Source: three-view drawing plus pictorial views. Frame: mm from the lowest corner of the part. A direction names the side the tool comes from. Coordinates: 2 decimals unless noted, no trailing zeros. Loops run counter-clockwise (first coordinate to the right, second up) from the corner with the lowest first, then second, coordinate; pieces in that order, holes last. Notation, with made-up numbers: (2, -27.5) - (52, -27.5) arc R22 ccw to (52, -3.5) - close; hole circle Ø2 at (-16.5, 44.5). An arc over 180 degrees is marked (long way). Return JSON: item names as keys, results as strings.
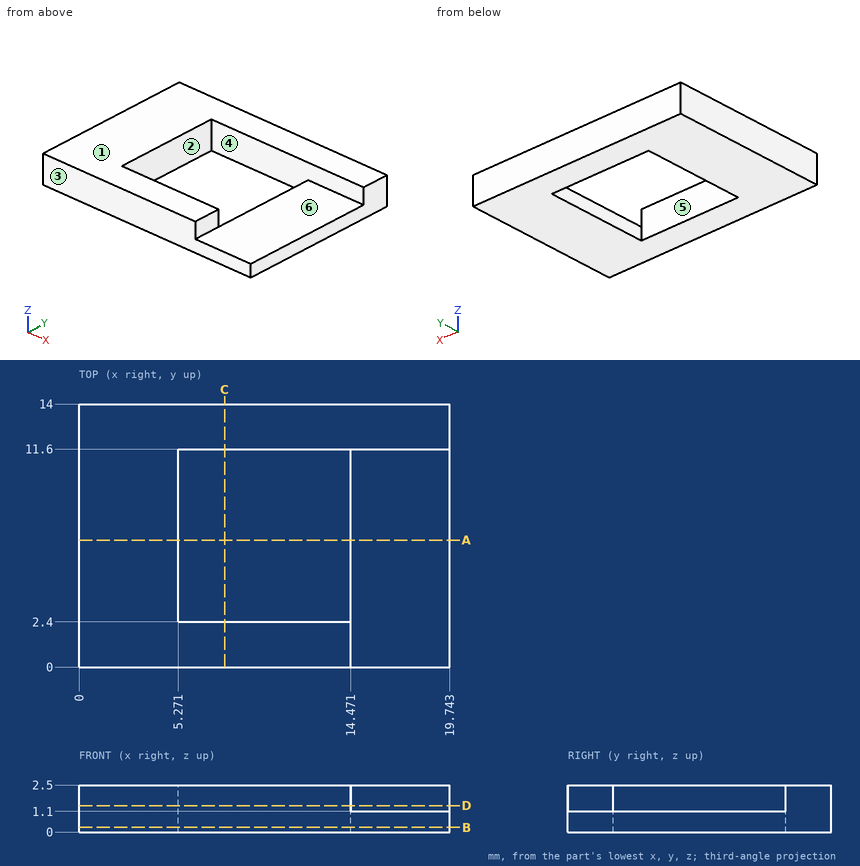
Item 1: First-contact query: pin 1 Ø1.6 at (x, y) = (16, 4.5) entering from +Z. Flat tip, straight axial feed; report the tip coordinate or a pass-through.
Worked out:
{"pin 1": "z = 1.1"}
Item 2: Reachability of the marked faces 4, 5 and 6 from +Z, -Z, +X, -X, +Y, -Y: full face, straight path, thin tool, end or side. Return the list, or none.
Worked out:
{"face 4": "+Z", "face 5": "+Z, -Z", "face 6": "+Z, +X, -Y"}
Item 3: Section query B-B, the plane z = 0.25. Return loops of the section in (x, y).
Worked out:
{"outline": "(0, 0) - (19.74, 0) - (19.74, 14) - (0, 14) - close; hole (5.27, 2.4) - (14.47, 2.4) - (14.47, 11.6) - (5.27, 11.6) - close"}
Item 4: Section query C-C, the plane x = 7.75. Return loops of the section in (y, z).
Worked out:
{"outline": "(0, 0) - (2.4, 0) - (2.4, 2.5) - (0, 2.5) - close; (11.6, 0) - (14, 0) - (14, 2.5) - (11.6, 2.5) - close"}
Item 5: Section query D-D, the plane z = 1.4. Return loops of the section in (x, y).
Worked out:
{"outline": "(0, 0) - (14.47, 0) - (14.47, 2.4) - (5.27, 2.4) - (5.27, 11.6) - (19.74, 11.6) - (19.74, 14) - (0, 14) - close"}
Item 6: Mould query, pull axis Y, two halves, no side actions, for the marked faces 1, 2 and 3. Classes: +Y half, -Y half, draft (parallel to the pull), parting line (faces both ways), or undercut.
Worked out:
{"face 1": "draft", "face 2": "undercut", "face 3": "-Y half"}
Item 7: Ray query, probe 1 along X at (y, z) = (4.5, 0.5); probe 2 along Y at (x, z) = (9.5, 2.15); probe 3 along X at (y, z) = (10.5, 2.2). Return the intervals inside material, ascending. Write a range as from..to.
Worked out:
{"probe 1": "0..5.27, 14.47..19.74", "probe 2": "0..2.4, 11.6..14", "probe 3": "0..5.27"}
Item 8: Section query A-A, the plane y = 6.75. Return loops of the section in (x, z), and give its area (3 significant figures).
Worked out:
{"outline": "(0, 0) - (5.27, 0) - (5.27, 2.5) - (0, 2.5) - close; (14.47, 0) - (19.74, 0) - (19.74, 1.1) - (14.47, 1.1) - close", "area": "19.0 mm^2"}
